Autodesk Inventor part; units mm, degrees
ref_plane "YZ Plane" through (0, 0, 0) normal (1, 0, 0) x (0, 1, 0)
ref_plane "XZ Plane" through (0, 0, 0) normal (0, 1, 0) x (-1, 0, 0)
ref_plane "XY Plane" through (0, 0, 0) normal (0, 0, 1) x (1, 0, 0)
sketch "Sketch1" plane through (0, 0, 0) normal (0, 0, 1) x (1, 0, 0)
  line L0 (-10, 0) -> (10, 0) construction
  line L1 (-10, -2.5) -> (10, -2.5)
  line L2 (10, 2.5) -> (-10, 2.5)
  arc A0 (-10, 2.5) -> (-10, -2.5) centre (-10, 0) ccw
  arc A1 (10, -2.5) -> (10, 2.5) centre (10, 0) ccw
  line L3 (17.5, 4.5) -> (17.5, -4.5)
  line L4 (-17.5, -4.5) -> (-17.5, 4.5)
  line L5 (-5, 70) -> (5, 70) construction
  line L6 (5, 70) -> (5, 8.5)
  line L7 (-5, 7.5) -> (-5, 7.5)
  line L8 (-5, 8.5) -> (-5, 70)
  line L9 (5, -7.5) -> (5, -7.5)
  line L10 (5, -8.5) -> (5, -42.5)
  line L11 (5, -42.5) -> (-5, -42.5) construction
  line L12 (-5, -42.5) -> (-5, -8.5)
  line L13 (14.5, -7.5) -> (6, -7.5)
  line L14 (-6, -7.5) -> (-14.5, -7.5)
  line L15 (-14.5, 7.5) -> (-6, 7.5)
  line L16 (6, 7.5) -> (14.5, 7.5)
  arc A2 (5, 70) -> (-5, 70) centre (0, 70) ccw
  circle A3 centre (0, 70) radius 1.5
  line L17 (0, 60) -> (0, 17.5) construction
  line L18 (-1.5, 60) -> (-1.5, 17.5)
  line L19 (1.5, 17.5) -> (1.5, 60)
  arc A4 (1.5, 60) -> (-1.5, 60) centre (0, 60) ccw
  arc A5 (-1.5, 17.5) -> (1.5, 17.5) centre (0, 17.5) ccw
  arc A6 (-5, -42.5) -> (5, -42.5) centre (0, -42.5) ccw construction
  line L20 (0, -42.5) -> (0, -17.5) construction
  line L21 (-1.5, -42.5) -> (-1.5, -17.5)
  line L22 (1.5, -17.5) -> (1.5, -42.5)
  arc A7 (-1.5, -42.5) -> (1.5, -42.5) centre (0, -42.5) ccw
  arc A8 (1.5, -17.5) -> (-1.5, -17.5) centre (0, -17.5) ccw
  arc A9 (17.5, 4.5) -> (14.5, 7.5) centre (14.5, 4.5) ccw
  arc A10 (14.5, -7.5) -> (17.5, -4.5) centre (14.5, -4.5) ccw
  arc A11 (-17.5, -4.5) -> (-14.5, -7.5) centre (-14.5, -4.5) ccw
  arc A12 (-14.5, 7.5) -> (-17.5, 4.5) centre (-14.5, 4.5) ccw
  arc A13 (-5, -8.5) -> (-6, -7.5) centre (-6, -8.5) ccw
  arc A14 (6, -7.5) -> (5, -8.5) centre (6, -8.5) ccw
  arc A15 (5, 8.5) -> (6, 7.5) centre (6, 8.5) ccw
  arc A16 (-6, 7.5) -> (-5, 8.5) centre (-6, 8.5) ccw
  line L23 (5, -42.5) -> (5, -46.5)
  line L24 (4, -47.5) -> (-4, -47.5)
  line L25 (-5, -46.5) -> (-5, -42.5)
  arc A17 (4, -47.5) -> (5, -46.5) centre (4, -46.5) ccw
  arc A18 (-5, -46.5) -> (-4, -47.5) centre (-4, -46.5) ccw
  point P0 (0, 0)
  point P1 (0, 2.5)
  point P2 (-17.5, 0)
  point P3 (17.5, 0)
  point P4 (0, 38.75)
  point P5 (0, -30)
  dimension "d0" = 10
  dimension "d1" = 35
  dimension "d2" = 15
  dimension "d3" = 5
  dimension "d4" = 20
  dimension "d5" = 3
  dimension "d6" = 10
  dimension "d7" = 10
  dimension "d8" = 70
  dimension "d9" = 3
  dimension "d10" = 35
  dimension "d11" = 3
  dimension "d12" = 10
  dimension "d13" = 3
  dimension "d14" = 1
  dimension "d17" = 1
extrude "Extrusion1" add sketch "Sketch1" against normal blind 3
properties part number "Slider_1"
Verification items for the finished model (mm, model axes). A direction names the side the tool comes from. Give positions to 0.01 mm unless a question says otherwise; leave off trailing zeros. Order: outer loops, then holes, each group sorted by start corner. A loop starts at its lowest first (then second) coordinate and runs counter-clockwise, first axis right, second up. Notation, with made-up numbers: M 87.5,89 L 128.5,89 A25 cw 128.5,124 Z; hole C 88,61.25 d9. An arc over 180 degrees is marked long. Return JSON: item names as keys, results as strings. Group by question number.
1) Section check A-A on x = 0. Record the cut outline in (y, z).
2) Scan lines: line 1 (Y direction, x = 0, z = -1.7); line 2 (Y direction, x = -8, z = -0.35); line 3 (X direction, y = 70, z = -1.35). Record each from-to range of solid material in increasing order.
3) Go/stop test with flat-tipped pins: pin 1 Ø0.9 at (x, z) = (-4.5, -2) entering from +Y; pin 2 Ø2.5 at (x, y) = (0, 70) entering from +Z; pin 3 Ø0.9 at (y, z) = (-22.5, -1) entering from +X; pin 4 Ø0.9 at (y, z) = (32, -1.5) entering from -X. Record where each tip stops, or that it passes through.
4) Section check C-C on y = -12. Record the cut outline in (x, z), and give its area (3 significant figures).
5) Section check B-B on x = 8.5. Record the cut outline in (y, z).
6) Access from +Z, -Z, +X, -X, +Y, -Y to the whole of each face (thin tool, end or side, straight path). Record for faces 1 (the face through (0, 16, -1)), 2 (the face through (10, -7.5, -1)), 3 (the face through (-10, -7.5, -1)), 4 (the face through (0, 75, -1)), 5 (the face through (17.5, 0, -1)).
7) Mould release check, pull along Y, two halves, no side actions. Record for faces 6 (the face through (10, 7.5, -1)), 7 (the face through (12.5, -0.1, -1.5)), 8 (the face through (-5, 39, -1)): pulls with the +Y half, pulls with the -Y half, needs draft (parallel to the pull), parting line crosses it, or undercut.
8) Section check D-D on z = -1.55. Give the number of separate pieces and of enclosed holes in the cut face, and give its area (3 significant figures).
Answer block:
{
 "1": {"outline": "M -47.5,-3 L -44,-3 L -44,0 L -47.5,0 Z; M -16,-3 L -2.5,-3 L -2.5,0 L -16,0 Z; M 2.5,-3 L 16,-3 L 16,0 L 2.5,0 Z; M 61.5,-3 L 68.5,-3 L 68.5,0 L 61.5,0 Z; M 71.5,-3 L 75,-3 L 75,0 L 71.5,0 Z"},
 "2": {"line 1": "y = -47.5 to -44, -16 to -2.5, 2.5 to 16, 61.5 to 68.5, 71.5 to 75", "line 2": "y = -7.5 to -2.5, 2.5 to 7.5", "line 3": "x = -5 to -1.5, 1.5 to 5"},
 "3": {"pin 1": "stops at y = 72.93", "pin 2": "passes through", "pin 3": "stops at x = 5", "pin 4": "stops at x = -5"},
 "4": {"outline": "M -5,-3 L 5,-3 L 5,0 L -5,0 Z", "area": "30.0 mm^2"},
 "5": {"outline": "M -7.5,-3 L -2.5,-3 L -2.5,0 L -7.5,0 Z; M 2.5,-3 L 7.5,-3 L 7.5,0 L 2.5,0 Z"},
 "6": {"face 1": "+Z, -Z", "face 2": "+Z, -Z, +X, -Y", "face 3": "+Z, -Z, -X, -Y", "face 4": "+Z, -Z, +Y", "face 5": "+Z, -Z, +X, +Y, -Y"},
 "7": {"face 6": "pulls with the +Y half", "face 7": "undercut", "face 8": "needs draft"},
 "8": {"separate pieces": "1", "enclosed holes": "4", "area": "1,240 mm^2"}
}
